Verification items for the finished model (mm, model axes). Face numbers are marked on the shaded views. Coordinates: 2 decimals unless noted, no trailing zeros. Order: outer loops, then holes, each group sorted by start corner. A loop starts at its lowest first (then second) coordinate and runs counter-clockwise, first axis right, second up. Notation, with made-up numbers: M 49.5,9.25 L 66.5,9.25 A18 ccw 66.5,34.25 Z; hole C -34.5,74 d4. An arc over 180 degrees is marked long. Return JSON: item names as keys, results as strings. Group by question number.
1. Section check A-A, the plane z = 20. Record the cut outline in (x, y).
2. Mould release check, pull along Y, two halves, no side actions. Record for the marked faces 1 and 2: +Y half, -Y half, draft (parallel to the pull), parting line (faces both ways), or undercut.
3. Material ranges on line 1 along Y through (x, z) = (0, 10.5); line 2 along Y through (x, z) = (2, 17); line 3 along X through (y, z) = (-4, 6), recorded low to high.
4. Section check B-B, the plane z = 28.5. Record the cut outline in (x, y), plus the area to 3 significant figures.
5. Gauge pin test, flat ends, axial feed: pin 1 (2 mm diameter, centred on y = 10, z = 6, fed in from +X); pin 2 (5 mm diameter, centred on x = -2.5, z = 21, fed in from -Y); pin 3 (10 mm diameter, centred on y = -5.5, z = 16.5, fed in from +X). Record the tip position at first contact, or that the pin passes through.
```python
from build123d import *

# Parameters (mm, degrees)
SKETCH001_R  = 13
SKETCH_R     = 12.5
SKETCH003_R  = 11.25
SKETCH002_R  = 11.25
CHAMFER_SIZE = 1


with BuildPart() as part:
    # Sketch001 (on DatumPlane) → AdditiveLoft section 0
    with BuildSketch(Plane.XY.offset(31)):
        Circle(SKETCH001_R)
    # Sketch → AdditiveLoft section 1
    with BuildSketch(Plane.XY):
        Circle(SKETCH_R)
    loft()

    # Sketch003 (on DatumPlane) → SubtractiveLoft section 0
    with BuildSketch(Plane.XY.offset(31)):
        Circle(SKETCH003_R)
    # Sketch002 → SubtractiveLoft section 1
    with BuildSketch(Plane.XY):
        Circle(SKETCH002_R)
    loft(mode=Mode.SUBTRACT)

    # Chamfer
    chamfer_edges = [part.edges().sort_by_distance(p)[0] for p in [
        (-12.5, 0, 0),
    ]]
    chamfer(chamfer_edges, length=CHAMFER_SIZE)


solid = part.part
```
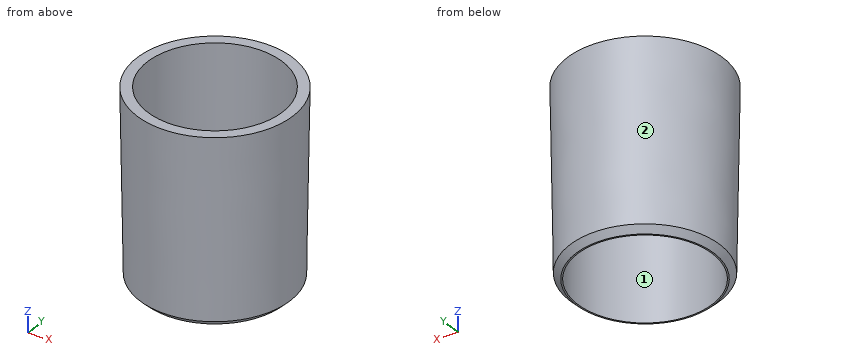
Answers follow:
{
 "1": {"outline": "C 0,0 d25.65; hole C 0,0 d22.5"},
 "2": {"face 1": "undercut", "face 2": "parting line"},
 "3": {"line 1": "-12.67 to -11.25, 11.25 to 12.67", "line 2": "-12.62 to -11.07, 11.07 to 12.62", "line 3": "-11.94 to -10.51, 10.51 to 11.94"},
 "4": {"outline": "C 0,0 d25.92; hole C 0,0 d22.5", "area": "130 mm^2"},
 "5": {"pin 1": "x = 8.81", "pin 2": "y = -12.85", "pin 3": "x = 12.77"}
}
